Could you check a few things on this model? Use its own coordinates, in mm. A direction names the side the tool comes from. Give positions to 0.01 mm unless a question says otherwise; leave off trailing zeros. Order: outer loops, then holes, each group sorted by start corner. A loop starts at its lowest first (then second) coordinate and runs counter-clockwise, first axis right, second up. Notation, with made-up numbers: (-10, 12) - (19, 12) arc R19 cw to (19, 47) - close; hole circle Ø10 at (-29.75, -18.5). An arc over 180 degrees is marked (long way). One line per question, with ' | ' between items. Start each with the question number.
1. For P1, Ø1, axis at x = 2, z = -11.5, coming from the -Y side; P2, Ø0.6, axis at x = 1.5, y = 2.5, coming from the -Z side; P3, Ø1.2, axis at x = -2, z = -9.5, coming from the +Y side, each with a flat end and sliding along its axis, tell me the tip position at first contact or that it passes through.
2. Imagine slicing it at A-A (y = -1.5). Please give me the cut outline in (x, z), and give its area (3 significant figures).
3. Which directions (+Z, -Z, +X, -X, +Y, -Y) give clear straight access to the entire face, cutting with the end or side of a thin tool? Please do faces 1 (the flat face through (1, -30, -14)), 2 (the flat face through (-2, 0, -28)), 3 (the flat face through (2, 30, -14)).
4. Imagine slicing it at B-B (z = -19.75). Please give me the cut outline in (x, y).
5. Imagine slicing it at C-C (x = 1.75). Please give me the cut outline in (y, z), and give its area (3 significant figures).
6. I need wall thicknesses on probe 1 along Z at (x, y) = (-2.1, -3); probe 2 along Y at (x, z) = (-1.05, -4). Which ranges of each line are inside material? Lowest first, please. Write a range as from..to.
```python
from build123d import *

# Parameters (mm, degrees)
F1_DEPTH = 28
F2_W     = 1.5
F2_H     = 66
F3_DEPTH = 2


with BuildPart() as f1:
    # F0 (on Top) → F1 (new body)
    with BuildSketch(Plane.XY):
        Polygon((0.5, -30), (2.5, -30), (2.5, 30), (0.5, 30), (-1, 30), (-2.5, 30), (-2.5, -30), (-1, -30), align=None)
        Polygon((-1, 30), (0.5, 30), (0.5, 31.5), (0.5, 33), (-1, 33), align=None)
        Polygon((0.5, -31.5), (0.5, -30), (-1, -30), (-1, -33), (0.5, -33), align=None)
    extrude(amount=-F1_DEPTH)

    # F2 (on face) → F3 (join)
    with BuildSketch(Plane(origin=(0, 0, -28), x_dir=(1, 0, 0), z_dir=(0, 0, -1))):
        with Locations((-0.25, 0)):
            Rectangle(F2_W, F2_H)
        Polygon((0.5, 30), (0.5, 33), (-1, 33), (-1, 30), (-1, -30), (-1, -33), (0.5, -33), (0.5, -30), align=None)
    extrude(amount=F3_DEPTH)


solid = f1.part
```
Results found:
1) P1: stops at y = -30 | P2: stops at z = -28 | P3: stops at y = 30
2) outline: (-2.5, -28) - (-1, -28) - (-1, -30) - (0.5, -30) - (0.5, -28) - (2.5, -28) - (2.5, 0) - (-2.5, 0) - close | area: 143 mm2
3) face 1: +Z, -Z, +X, -Y | face 2: -Z, -X, +Y, -Y | face 3: +Z, -Z, +X, +Y
4) outline: (-2.5, -30) - (-1, -30) - (-1, -33) - (0.5, -33) - (0.5, -30) - (2.5, -30) - (2.5, 30) - (0.5, 30) - (0.5, 33) - (-1, 33) - (-1, 30) - (-2.5, 30) - close
5) outline: (-30, -28) - (30, -28) - (30, 0) - (-30, 0) - close | area: 1,680 mm2
6) probe 1: z = -28..0 | probe 2: y = -30..30
